from build123d import *

# Parameters (mm, degrees)
F0_W     = 195.8933323622
F0_H     = 92.163823545
F1_DEPTH = 25.4
F2_R     = 6.35
F3_DEPTH = 25.4
F4_W     = 36.7853008211
F4_H     = 33.6875878274
F6_W     = 25.4169069231
F6_H     = 12.7084553242


with BuildPart() as f1:
    # F0 (on Top) → F1 (new body)
    with BuildSketch(Plane.XY):
        Rectangle(F0_W, F0_H)
    extrude(amount=F1_DEPTH)

    # F2 (on Top) → F3 (cut)
    with BuildSketch(Plane.XY):
        with Locations((-85.2466661811, 33.3819117725)):
            Circle(F2_R)
        with Locations((-85.2466661811, -33.3819117725)):
            Circle(F2_R)
        with Locations((85.2466661811, 33.3819117725)):
            Circle(F2_R)
        with Locations((85.2466661811, -33.3819117725)):
            Circle(F2_R)
    extrude(amount=F3_DEPTH, mode=Mode.SUBTRACT)

    # F4 (on Front) → F5 (revolve)
    with BuildSketch(Plane.XZ):
        with Locations((-18.3926504105, 42.2437939137)):
            Rectangle(F4_W, F4_H)
    revolve(axis=Axis((0, 0, 42.2437939137), (0, 0, -1)))

    # F6 (on Front) → F7 (revolve, cut)
    with BuildSketch(Plane.XZ):
        with Locations((-39.2806772143, 40.7248176634)):
            Rectangle(F6_W, F6_H)
    revolve(axis=Axis((0, 0, 59.0875878274), (0, 0, -1)), mode=Mode.SUBTRACT)


solid = f1.part
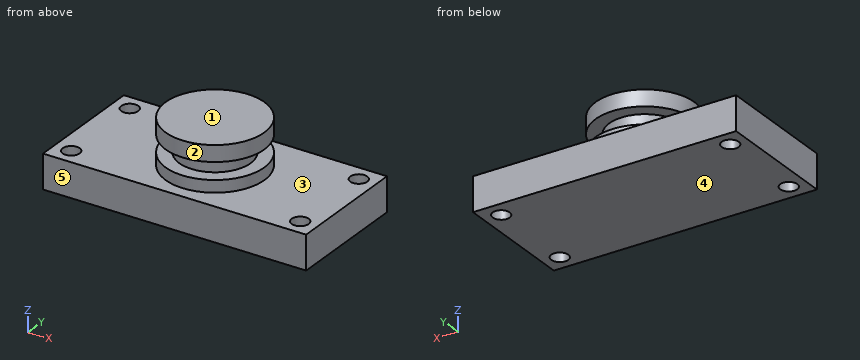
Input: part model. Units: mm. Frame: model coordinates. Face numbers are marked on the shaded views. A direction names the side the tool comes from. Coordinates: 2 decimals unless noted, no trailing zeros. Loops run counter-clockwise (first coordinate to the right, second up) from the corner with the lowest first, then second, coordinate; pieces in that order, holes last. Notation, with made-up numbers: (38.5, 0) - (97.5, 0) arc R20 cw to (97.5, 13) - close; hole circle Ø8 at (-27, 55). An arc over 180 degrees is marked (long way). Answer in a Markdown table with one row per item. Add a question column.
Item 1: Section query D-D on z = 23.5. Return the cut outline in (x, y), then the cut area to 3 significant figures.
Item 2: Section query B-B on y = 0. Return the cut outline in (x, z).
Item 3: Mould query, pull axis Z, two halves, no side actions, for the marked faces 3, 4 and 5. Classes: released by +Z, released by -Z, zero draft, split by the parting line, or undercut.
Item 4: Line query: line 1 along Y through (x, z) = (83, 6); line 2 along X through (y, z) = (36, 5); line 3 along X through (y, z) = (38.5, 10.5). Output: solid intervals per line, ascending. Write a range as [from, to].
Item 5: Section query C-C on y = 30. Return the cut outline in (x, z), then the cut area to 3 significant figures.
Item 6: Section query A-A on x = 0. Return the cut outline in (y, z).
Item 7: Contact query for flat-ended pins moving along their axis: P1, Ø10, axis at x = -85.25, y = 33.38, coming from the +Z side; P2, Ø3, axis at y = 1, z = 33, coming from the +X side; P3, Ø20.5, axis at x = -85.25, y = -33.38, coming from the +Z side. Output: stop coordinate, or through.
Item 8: Access query for the marked faces 1 and 2. Directions: +Z, -Z, +X, -X, +Y, -Y. A direction counts if a zero-diameter tool reaches every point of the face in a straight line with its end or side. Return the directions, or none.
Recorded:
| question | item | result |
|---|---|---|
| 1 | outline | (-97.95, -46.08) - (97.95, -46.08) - (97.95, 46.08) - (-97.95, 46.08) - close; hole circle Ø12.7 at (-85.25, -33.38); hole circle Ø12.7 at (-85.25, 33.38); hole circle Ø12.7 at (85.25, -33.38); hole circle Ø12.7 at (85.25, 33.38) |
| 1 | area | 17,500 mm^2 |
| 2 | outline | (-97.95, 0) - (97.95, 0) - (97.95, 25.4) - (36.79, 25.4) - (36.79, 34.37) - (26.57, 34.37) - (26.57, 47.08) - (36.79, 47.08) - (36.79, 59.09) - (-36.79, 59.09) - (-36.79, 47.08) - (-26.57, 47.08) - (-26.57, 34.37) - (-36.79, 34.37) - (-36.79, 25.4) - (-97.95, 25.4) - close |
| 3 | face 3 | released by +Z |
| 3 | face 4 | released by -Z |
| 3 | face 5 | zero draft |
| 4 | line 1 | [-46.08, -39.32], [-27.44, 27.44], [39.32, 46.08] |
| 4 | line 2 | [-97.95, -91.03], [-79.46, 79.46], [91.03, 97.95] |
| 4 | line 3 | [-97.95, -89.01], [-81.49, 81.49], [89.01, 97.95] |
| 5 | outline | (-97.95, 0) - (-90.62, 0) - (-90.62, 25.4) - (-97.95, 25.4) - close; (-79.87, 0) - (79.87, 0) - (79.87, 25.4) - (21.29, 25.4) - (21.29, 34.37) - (-21.29, 34.37) - (-21.29, 25.4) - (-79.87, 25.4) - close; (-21.29, 47.08) - (21.29, 47.08) - (21.29, 59.09) - (-21.29, 59.09) - close; (90.62, 0) - (97.95, 0) - (97.95, 25.4) - (90.62, 25.4) - close |
| 5 | area | 5,320 mm^2 |
| 6 | outline | (-46.08, 0) - (46.08, 0) - (46.08, 25.4) - (36.79, 25.4) - (36.79, 34.37) - (26.57, 34.37) - (26.57, 47.08) - (36.79, 47.08) - (36.79, 59.09) - (-36.79, 59.09) - (-36.79, 47.08) - (-26.57, 47.08) - (-26.57, 34.37) - (-36.79, 34.37) - (-36.79, 25.4) - (-46.08, 25.4) - close |
| 7 | P1 | through |
| 7 | P2 | x = 36.79 |
| 7 | P3 | z = 25.4 |
| 8 | face 1 | +Z, +X, -X, +Y, -Y |
| 8 | face 2 | +Z |
